Part model, mm, in its own coordinate system. Give positions to 0.01 mm unless a question says otherwise; leave off trailing zeros. One line per question, with ' | ' between items.
```python
from build123d import *

# Parameters (mm, degrees)
F0_W          = 555
F0_H          = 355
F1_DEPTH      = 2.5
F2_R          = 9.5
F3_DEPTH      = 2.501
F3_DEPTH_BACK = 2.501


with BuildPart() as f1:
    # F0 (on Front) → F1 (new body, symmetric)
    with BuildSketch(Plane.XZ):
        Rectangle(F0_W, F0_H)
    extrude(amount=F1_DEPTH, both=True)

    # F2 (on Front) → F3 (cut, two sides)
    with BuildSketch(Plane.XZ) as f3_sk:
        with Locations((-240, -140)):
            Circle(F2_R)
        with Locations((-240, -100)):
            Circle(F2_R)
        with Locations((-240, -60)):
            Circle(F2_R)
        with Locations((-120, -140)):
            Circle(F2_R)
        with Locations((-120, -100)):
            Circle(F2_R)
        with Locations((-120, -60)):
            Circle(F2_R)
        with Locations((-80, -140)):
            Circle(F2_R)
        with Locations((-80, -100)):
            Circle(F2_R)
        with Locations((-80, -60)):
            Circle(F2_R)
        with Locations((-240, -20)):
            Circle(F2_R)
        with Locations((-120, -20)):
            Circle(F2_R)
        with Locations((-80, -20)):
            Circle(F2_R)
        with Locations((-40, -140)):
            Circle(F2_R)
        with Locations((-40, -100)):
            Circle(F2_R)
        with Locations((-40, -60)):
            Circle(F2_R)
        with Locations((-40, -20)):
            Circle(F2_R)
        with Locations((0, -140)):
            Circle(F2_R)
        with Locations((0, -100)):
            Circle(F2_R)
        with Locations((0, -60)):
            Circle(F2_R)
        with Locations((0, -20)):
            Circle(F2_R)
        with Locations((40, -140)):
            Circle(F2_R)
        with Locations((40, -100)):
            Circle(F2_R)
        with Locations((40, -60)):
            Circle(F2_R)
        with Locations((40, -20)):
            Circle(F2_R)
        with Locations((80, -140)):
            Circle(F2_R)
        with Locations((80, -100)):
            Circle(F2_R)
        with Locations((80, -60)):
            Circle(F2_R)
        with Locations((80, -20)):
            Circle(F2_R)
        with Locations((120, -140)):
            Circle(F2_R)
        with Locations((120, -100)):
            Circle(F2_R)
        with Locations((120, -60)):
            Circle(F2_R)
        with Locations((120, -20)):
            Circle(F2_R)
        with Locations((-240, 20)):
            Circle(F2_R)
        with Locations((-240, 60)):
            Circle(F2_R)
        with Locations((-240, 100)):
            Circle(F2_R)
        with Locations((-240, 140)):
            Circle(F2_R)
        with Locations((-120, 20)):
            Circle(F2_R)
        with Locations((-120, 60)):
            Circle(F2_R)
        with Locations((-120, 100)):
            Circle(F2_R)
        with Locations((-120, 140)):
            Circle(F2_R)
        with Locations((-80, 20)):
            Circle(F2_R)
        with Locations((-80, 60)):
            Circle(F2_R)
        with Locations((-80, 100)):
            Circle(F2_R)
        with Locations((-80, 140)):
            Circle(F2_R)
        with Locations((-40, 20)):
            Circle(F2_R)
        with Locations((-40, 60)):
            Circle(F2_R)
        with Locations((-40, 100)):
            Circle(F2_R)
        with Locations((-40, 140)):
            Circle(F2_R)
        with Locations((0, 20)):
            Circle(F2_R)
        with Locations((0, 60)):
            Circle(F2_R)
        with Locations((0, 100)):
            Circle(F2_R)
        with Locations((0, 140)):
            Circle(F2_R)
        with Locations((40, 20)):
            Circle(F2_R)
        with Locations((40, 60)):
            Circle(F2_R)
        with Locations((40, 100)):
            Circle(F2_R)
        with Locations((40, 140)):
            Circle(F2_R)
        with Locations((80, 20)):
            Circle(F2_R)
        with Locations((80, 60)):
            Circle(F2_R)
        with Locations((80, 100)):
            Circle(F2_R)
        with Locations((80, 140)):
            Circle(F2_R)
        with Locations((120, 20)):
            Circle(F2_R)
        with Locations((120, 60)):
            Circle(F2_R)
        with Locations((120, 100)):
            Circle(F2_R)
        with Locations((120, 140)):
            Circle(F2_R)
        with Locations((240, -140)):
            Circle(F2_R)
        with Locations((240, -100)):
            Circle(F2_R)
        with Locations((240, -60)):
            Circle(F2_R)
        with Locations((240, -20)):
            Circle(F2_R)
        with Locations((240, 20)):
            Circle(F2_R)
        with Locations((240, 60)):
            Circle(F2_R)
        with Locations((240, 100)):
            Circle(F2_R)
        with Locations((240, 140)):
            Circle(F2_R)
    extrude(amount=F3_DEPTH, mode=Mode.SUBTRACT)
    extrude(f3_sk.sketch, amount=-F3_DEPTH_BACK, mode=Mode.SUBTRACT)


solid = f1.part
```
1. Drop a flat-ended pin along its axis: pin 1 (15 mm diameter, centred on x = 120, z = 20, fed in from -Y). Give the stop position or say it passes through.
Worked out:
pin 1: passes through
2. Mould opens along X. For faces 1 (the flat face through (-4, 2.5, 2)), 2 (the cylindrical face through (-122.059, -0.035, 130.726)) say: released by +X, released by -X, zero draft, split by the parting line, or undercut.
Worked out:
face 1: zero draft | face 2: undercut
3. Slice it at A-A on x = 0. Give the number of separate pieces and of enclosed holes in the cut face, then the cut area to 4 significant figures.
Worked out:
separate pieces: 9 | enclosed holes: 0 | area: 1,015 mm2
